Could you check a few things on this model? Use its own coordinates, in mm. Face numbers are marked on the shaded views. Coordinates: 2 decimals unless noted, no trailing zeros. Loops run counter-clockwise (first coordinate to the right, second up) from the corner with the lowest first, then second, coordinate; pieces in that order, holes last. Notation, with made-up numbers: (60.5, -25.75) -> (81.5, -25.75) arc R27 cw to (81.5, 2.25) -> close; hole circle Ø10 at (89.5, 18). An arc over 180 degrees is marked (long way). One line per question, with ' | ' between items. Start each with the question number.
(1) Suppose I cut it at B-B (x = 100). Please give me the cut outline in (y, z), plus the area to 3 significant figures.
(2) Suppose I cut it at C-C (x = 103.5). Please give me the cut outline in (y, z).
(3) If I drill on line 1 along Y through (x, z) = (105, 1); line 2 along X through (y, z) = (-302.25, 0.6); line 3 along X through (y, z) = (-301.5, 3.75), over which ranges is the centre line in solid material (lowest first)?
(4) Suppose I cut it at A-A (y = -307.75). Please give me the cut outline in (x, z), plus the area to 3 significant figures.
(5) If we mould it in two halves opening along X, with no side actions, what happens to the marked faces 1, 2, 3 and 4? For each: pulls with the +X half, pulls with the -X half, needs draft (parallel to the pull), parting line crosses it, or undercut.
(6) I'm going to push flat-ended pins straight in: pin 1 Ø2 at (y, z) = (-311.5, 3.5) entering from +X; pin 2 Ø2 at (y, z) = (-298.5, 3.5) entering from -X; pin 3 Ø3 at (x, y) = (111.61, -302.77) entering from +Z. Where does each tip first touch, or does it pass through?
(7) Suppose I cut it at D-D (z = 3.4). Please give me the cut outline in (x, y), plus the area to 3 significant figures.
```python
from build123d import *

# Parameters (mm, degrees)
RESSALTO_EXTRUS_O1_DEPTH = 4
ESBO_O2_R                = 5.25
CORTE_EXTRUS_O1_DEPTH    = 4
M3_CLEARANCE_HOLE1_D     = 3.2


with BuildPart() as part:
    # Esboço1 → Ressalto-extrusão1 (new body)
    with BuildSketch(Plane.XY):
        with BuildLine():
            Line((95.202808527, -295.7159332), (112.09037792, -295.7159332))
            ThreePointArc((112.09037792, -295.7159332), (103.646593224, -313.7659332), (95.202808527, -295.7159332))
        make_face()
    extrude(amount=RESSALTO_EXTRUS_O1_DEPTH)

    # Esboço2 → Corte-extrusão1 (cut)
    with BuildSketch(Plane.XY.offset(4)):
        with Locations((103.646593224, -302.7659332)):
            Circle(ESBO_O2_R)
    extrude(amount=-CORTE_EXTRUS_O1_DEPTH, mode=Mode.SUBTRACT)

    # M3 Clearance Hole1 (through all)
    with Locations(Plane.XY.offset(4)):
        with Locations((95.681870132, -302.765933199), (111.611316315, -302.765933199), (103.646593224, -310.730656291), (103.646593224, -294.801210108)):
            Hole(M3_CLEARANCE_HOLE1_D / 2)


solid = part.part
```
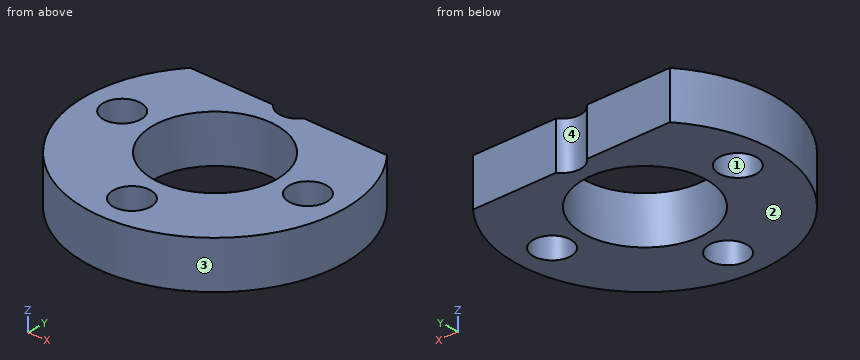
Checks:
1) outline: (-313.14, 0) -> (-306.54, 0) -> (-306.54, 4) -> (-313.14, 4) -> close; (-298.99, 0) -> (-295.72, 0) -> (-295.72, 4) -> (-298.99, 4) -> close | area: 39.5 mm^2
2) outline: (-313.76, 0) -> (-312.32, 0) -> (-312.32, 4) -> (-313.76, 4) -> close; (-309.14, 0) -> (-308.01, 0) -> (-308.01, 4) -> (-309.14, 4) -> close; (-297.52, 0) -> (-296.39, 0) -> (-296.39, 4) -> (-297.52, 4) -> close
3) line 1: y = -313.68 to -311.58, -309.88 to -307.84, -297.69 to -295.72 | line 2: x = 92.66 to 94.17, 97.2 to 98.42, 108.87 to 110.1, 113.13 to 114.63 | line 3: x = 92.72 to 94.7, 96.66 to 98.55, 108.74 to 110.63, 112.59 to 114.57
4) outline: (93.84, 0) -> (102, 0) -> (102, 4) -> (93.84, 4) -> close; (105.3, 0) -> (113.45, 0) -> (113.45, 4) -> (105.3, 4) -> close | area: 65.3 mm^2
5) face 1: undercut | face 2: needs draft | face 3: parting line crosses it | face 4: undercut
6) pin 1: stops at x = 111.47 | pin 2: stops at x = 93.14 | pin 3: passes through
7) outline: (95.2, -295.72) arc R11 ccw (long way) to (112.09, -295.72) -> (104.96, -295.72) arc R1.6 cw to (102.33, -295.72) -> close; hole circle Ø3.2 at (95.68, -302.77); hole circle Ø10.5 at (103.65, -302.77); hole circle Ø3.2 at (103.65, -310.73); hole circle Ø3.2 at (111.61, -302.77) | area: 222 mm^2
